The model under review builds one solid part; all positions refer to its coordinate system, in mm. Face numbers are marked on the shaded views. A direction names the side the tool comes from. Coordinates: 2 decimals unless noted, no trailing zeros. Order: outer loops, then holes, each group sorted by start corner. A loop starts at its lowest first (then second) coordinate and runs counter-clockwise, first axis right, second up. Notation, with made-up numbers: (-39.75, 70) - (19.25, 70) arc R26 ccw to (19.25, 103) - close; hole circle Ø7 at (-14.75, -24). An arc over 180 degrees is marked (long way). Answer in a Markdown table with one row per item.
```python
from build123d import *

# Parameters (mm, degrees)
BOSS_EXTRUDE1_DEPTH = 15.24
SKETCH2_R           = 6
BOSS_EXTRUDE2_DEPTH = 5.08
FILLET1_R           = 0.254


with BuildPart() as part:
    # Sketch1 → Boss-Extrude1 (new body)
    with BuildSketch(Plane(origin=(0, 0, 0), x_dir=(1, 0, 0), z_dir=(0, 1, 0))):
        with BuildLine():
            Line((-1.658312395, 2.5), (1.658312395, 2.5))
            ThreePointArc((1.658312395, 2.5), (0, -3), (-1.658312395, 2.5))
        make_face()
    extrude(amount=BOSS_EXTRUDE1_DEPTH)

    # Sketch2 → Boss-Extrude2 (add)
    with BuildSketch(Plane(origin=(0, 15.24, 0), x_dir=(1, 0, 0), z_dir=(0, 1, 0))):
        Circle(SKETCH2_R)
    extrude(amount=BOSS_EXTRUDE2_DEPTH)

    # Fillet1
    fillet1_edges = [part.edges().sort_by_distance(p)[0] for p in [
        (0, 0, 3),
    ]]
    fillet(fillet1_edges, radius=FILLET1_R)


solid = part.part
```
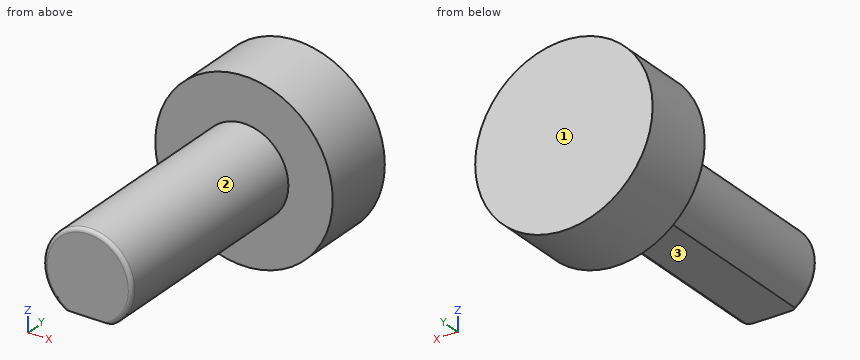
Item 1: We need section C-C, the plane y = 16.25. Write out the cut boundary in (x, z).
Check values:
| item | result |
|---|---|
| outline | circle Ø12 at (0, 0) |
Item 2: We need section A-A, the plane x = 0. Write out the cut boundary in (y, z).
Check values:
| item | result |
|---|---|
| outline | (0, -2.5) - (15.24, -2.5) - (15.24, -6) - (20.32, -6) - (20.32, 6) - (15.24, 6) - (15.24, 3) - (0.25, 3) arc R0.25 ccw to (0, 2.75) - close |
Item 3: Clearance check with flat-ended pins moving along their axes: pin 1 Ø1 at (y, z) = (6, 0) entering from -X; pin 2 Ø3 at (x, y) = (0.5, 7) entering from -Z; pin 3 Ø5 at (y, z) = (14, -0.5) entering from +X; pin 4 Ø1 at (y, z) = (7.5, 4) entering from -X. State where each tip first meets the part, or that it passes through.
Check values:
| item | result |
|---|---|
| pin 1 | x = -3 |
| pin 2 | z = -2.5 |
| pin 3 | x = 6 |
| pin 4 | through |
Item 4: We need section D-D, the plane x = 3.75. Write out the cut boundary in (y, z).
Check values:
| item | result |
|---|---|
| outline | (15.24, -4.68) - (20.32, -4.68) - (20.32, 4.68) - (15.24, 4.68) - close |
Item 5: To check wall thickness, follow line 1 (Y direction, x = -3.75, z = 1.5); line 2 (Z direction, x = -2.5, y = 5.75); line 3 (X direction, y = 18.25, z = -5). State the ranges of each line that lie inside material, in increasing order. Write a range as from..to.
Check values:
| item | result |
|---|---|
| line 1 | 15.24..20.32 |
| line 2 | -1.66..1.66 |
| line 3 | -3.32..3.32 |
Item 6: We need section B-B, the plane y = 3.75. Write out the cut boundary in (x, z), then the cut area to 3 significant figures.
Check values:
| item | result |
|---|---|
| outline | (-1.66, -2.5) - (1.66, -2.5) arc R3 ccw (long way) to start |
| area | 27.1 mm^2 |
Item 7: Tool access review of the marked faces 1, 2 and 3: name each direction out of +Z, -Z, +X, -X, +Y, -Y from which nothing blocks a thin tool from reaching the whole face with its end or side.
Check values:
| item | result |
|---|---|
| face 1 | +Z, -Z, +X, -X, +Y |
| face 2 | -Y |
| face 3 | -Z, +X, -X, -Y |
